from build123d import *

# Parameters (mm, degrees)
SKETCH1_W           = 70
SKETCH1_H           = 55
SKETCH1_W_2         = 150
SKETCH1_H_2         = 82
BOSS_EXTRUDE1_DEPTH = 6
SKETCH2_W           = 6
SKETCH2_H           = 10
CUT_EXTRUDE1_DEPTH  = 10
SKETCH3_R           = 1.5
CUT_EXTRUDE2_DEPTH  = 6
SKETCH4_W           = 25
SKETCH4_H           = 6
CUT_EXTRUDE3_DEPTH  = 6


with BuildPart() as part:
    # Sketch1 → Boss-Extrude1 (new body)
    with BuildSketch(Plane.XY):
        with Locations((0, -68.5)):
            Rectangle(SKETCH1_W, SKETCH1_H)
        Rectangle(SKETCH1_W_2, SKETCH1_H_2)
    extrude(amount=BOSS_EXTRUDE1_DEPTH)

    # Sketch2 → Cut-Extrude1 (cut)
    with BuildSketch(Plane.XY.offset(6)):
        with Locations((-72, 30)):
            Rectangle(SKETCH2_W, SKETCH2_H)
        with Locations((72, 30)):
            Rectangle(SKETCH2_W, SKETCH2_H)
        with Locations((72, 10)):
            Rectangle(SKETCH2_W, SKETCH2_H)
        with Locations((-72, 10)):
            Rectangle(SKETCH2_W, SKETCH2_H)
        with Locations((-72, -10)):
            Rectangle(SKETCH2_W, SKETCH2_H)
        with Locations((72, -10)):
            Rectangle(SKETCH2_W, SKETCH2_H)
        with Locations((-72, -30)):
            Rectangle(SKETCH2_W, SKETCH2_H)
        with Locations((72, -30)):
            Rectangle(SKETCH2_W, SKETCH2_H)
    extrude(amount=-CUT_EXTRUDE1_DEPTH, mode=Mode.SUBTRACT)

    # Sketch3 → Cut-Extrude2 (cut)
    with BuildSketch(Plane.XY.offset(6)):
        with Locations((-29, 1)):
            Circle(SKETCH3_R)
        with Locations(Location((29, 1, 0), (0, 0, 180))):
            Circle(SKETCH3_R)
        with BuildLine():
            Line((-9, 1), (-24, 1))
            ThreePointArc((-24, 1), (-32.535533906, -2.535533906), (-29, 6))
            Line((-29, 6), (-29, 21))
            ThreePointArc((-29, 21), (-43.142135624, -13.142135624), (-9, 1))
        make_face()
        with BuildLine():
            Line((9, 1), (24, 1))
            ThreePointArc((24, 1), (32.535533906, -2.535533906), (29, 6))
            Line((29, 6), (29, 21))
            ThreePointArc((29, 21), (43.142135624, -13.142135624), (9, 1))
        make_face()
    extrude(amount=-CUT_EXTRUDE2_DEPTH, mode=Mode.SUBTRACT)

    # Sketch4 → Cut-Extrude3 (cut)
    with BuildSketch(Plane.XY.offset(6)):
        with Locations((12.5, 38)):
            Rectangle(SKETCH4_W, SKETCH4_H)
        with Locations((62.5, 38)):
            Rectangle(SKETCH4_W, SKETCH4_H)
        with Locations((-37.5, 38)):
            Rectangle(SKETCH4_W, SKETCH4_H)
    extrude(amount=-CUT_EXTRUDE3_DEPTH, mode=Mode.SUBTRACT)


solid = part.part
Could you check a few things on this model? Use its own coordinates, in mm. A direction names the side the tool comes from. Coordinates: 2 decimals unless noted, no trailing zeros. Loops run counter-clockwise (first coordinate to the right, second up) from the corner with the lowest first, then second, coordinate; pieces in that order, holes last.
1. Imagine slicing it at A-A (y = 11.5). Please give me the cut outline in (x, z).
2. We'd pull the mould along X, two halves only. Please class faces 5 (the face through (-1, -27, 0)), 6 (the face through (-75, 38, 3)), 7 (the face through (16, 1, 3)): released by +X, released by -X, zero draft, split by the parting line, or undercut.
3. For P1, Ø1.5, axis at y = -46.5, z = 2, coming from the -X side; P2, Ø3, axis at y = 39, z = 3.5, coming from the +X side; P3, Ø3, axis at y = -31.5, z = 2, coming from the -X side, each with a flat end and sliding along its axis, tell me the tip position at first contact or that it passes through.
4. Imagine slicing it at C-C (y = -55). Please give me the cut outline in (x, z), and give its area (3 significant figures).
5. I need wall thicknesses on L1, parallel to X at y = 8, z = 1.9 (3 decimals); L2, parallel to Y at x = 33.5, z = 1.95; L3, parallel to Y at x = -64, z = 3.9. Which ranges of each line are inside material? Lowest first, please.
6. Imagine slicing it at B-B (z = 2.3). Give the number of separate pieces and of enclosed holes in the cut face, and give its area (3 significant figures).
7. For faces 1 (the face through (-55, -41, 3)), 2 (the face through (-72, -25, 3)), 3 (the face through (59, 35, 3)), 4 (the face through (72, -15, 3)), which set-ups out of +Z, -Z, +X, -X, +Y, -Y let a thin tool reach every point of the face, with its end or its side?
Computed values:
1. outline: (-69, 0) - (-46.02, 0) - (-46.02, 6) - (-69, 6) - close; (-29, 0) - (29, 0) - (29, 6) - (-29, 6) - close; (46.02, 0) - (69, 0) - (69, 6) - (46.02, 6) - close
2. face 5: zero draft
2. face 6: released by -X
2. face 7: undercut
3. P1: stops at x = -35
3. P2: stops at x = 50
3. P3: stops at x = -69
4. outline: (-35, 0) - (35, 0) - (35, 6) - (-35, 6) - close
4. area: 420 mm2
5. L1: x = -69 to -47.735, -29 to 29, 47.735 to 69
5. L2: y = -96 to -18.49, -1.18 to 3.18, 20.49 to 41
5. L3: y = -41 to 41
6. separate pieces: 1
6. enclosed holes: 4
6. area: 13,400 mm2
7. face 1: +Z, -Z, -X, -Y
7. face 2: +Z, -Z, -X
7. face 3: +Z, -Z, +X, +Y
7. face 4: +Z, -Z, +X
